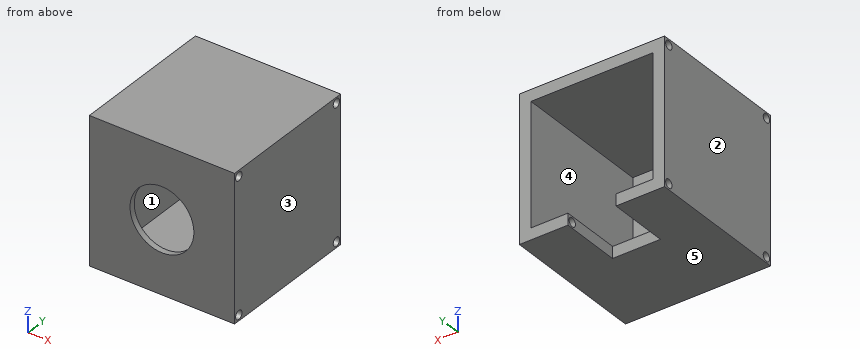
Autodesk Inventor part; units mm, degrees
ref_plane "YZ Plane" through (0, 0, 0) normal (1, 0, 0) x (0, 1, 0)
ref_plane "XZ Plane" through (0, 0, 0) normal (0, 1, 0) x (-1, 0, 0)
ref_plane "XY Plane" through (0, 0, 0) normal (0, 0, 1) x (1, 0, 0)
sketch "Sketch1" plane through (0, 0, 0) normal (0, 0, 1) x (1, 0, 0)
  line L0 (-25, -25) -> (25, -25)
  line L1 (25, -25) -> (25, 25)
  line L2 (25, 25) -> (-25, 25)
  line L3 (-25, 25) -> (-25, -25)
  line L4 (-25, -25) -> (25, 25) construction
  line L5 (25, -25) -> (-25, 25) construction
  point P0 (0, 0)
  dimension "d0" = 50
  dimension "d1" = 50
extrude "Main Block" add sketch "Sketch1" along normal blind 50
sketch "Sketch2" plane through (-25, 25, 0) normal (0, 1, 0) x (1, 0, 0)
  line L0 (0, -50) -> (50, -50) construction
  line L1 (0, 0) -> (50, 0) construction
  line L2 (50, -50) -> (0, 0) construction
  line L3 (46, -46) -> (4, -46)
  line L4 (4, -46) -> (4, -4)
  line L5 (4, -4) -> (46, -4)
  line L6 (46, -4) -> (46, -46)
  line L7 (46, -46) -> (4, -4) construction
  line L8 (4, -46) -> (46, -4) construction
  line L9 (25, -25) -> (25, -46) construction
  point P0 (25, 0)
  dimension "d4" = 42
  dimension "d5" = 42
extrude "Motor Void" cut sketch "Sketch2" against normal blind 48
sketch "Sketch3" plane through (-25, 25, 0) normal (0, 1, 0) x (1, 0, 0)
  line L0 (25, 0) -> (25, -4) construction
  line L1 (4, -4) -> (46, -4) construction
  line L2 (16.75, -4) -> (33.25, -4)
  line L3 (33.25, -4) -> (33.25, 0)
  line L4 (33.25, 0) -> (16.75, 0)
  line L5 (16.75, 0) -> (16.75, -4)
  line L6 (16.75, -4) -> (33.25, 0) construction
  line L7 (33.25, -4) -> (16.75, 0) construction
  point P0 (25, -2)
  dimension "d8" = 16.5
  dimension "d9" = 4
extrude "Cable Void" cut sketch "Sketch3" against normal blind 21
sketch "Sketch4" plane through (-25, -25, 0) normal (0, -1, 0) x (1, 0, 0)
  line L0 (0, 0) -> (0, 50) construction
  line L1 (50, 50) -> (0, 50) construction
  line L2 (0, 0) -> (50, 50) construction
  circle A0 centre (25, 25) radius 11
  point P0 (25, 0)
  dimension "d12" = 22
extrude "Raised Void" cut sketch "Sketch4" against normal blind 2
sketch "Sketch5" plane through (-25, -25, 0) normal (-1, 0, 0) x (0, 0, 1)
  line L0 (0, 0) -> (0, 50) construction
  line L1 (4, 50) -> (4, 2) construction
  line L2 (0, 50) -> (4, 50) construction
  line L3 (0, 50) -> (50, 50) construction
  line L4 (46, 2) -> (4, 2) construction
  line L5 (4, 50) -> (4, 2) construction
  line L6 (4, 2) -> (46, 2) construction
  line L7 (46, 50) -> (46, 2) construction
  line L8 (46, 2) -> (46, 50) construction
  line L9 (50, 0) -> (50, 50) construction
  line L10 (46, 50) -> (50, 50) construction
  line L11 (50, 50) -> (48, 50) construction
  line L12 (48, 50) -> (48, 48) construction
  circle A0 centre (48, 48) radius 1.5
  line L13 (48, 0) -> (48, 2) construction
  line L14 (48, 0) -> (50, 0) construction
  line L15 (0, 50) -> (4, 50) construction
  line L16 (2, 50) -> (2, 48) construction
  line L17 (0, 0) -> (50, 0) construction
  line L18 (2, 0) -> (2, 2) construction
  line L19 (2, 0) -> (4, 0) construction
  circle A1 centre (2, 48) radius 1.5
  circle A2 centre (2, 2) radius 1.5
  circle A3 centre (48, 2) radius 1.5
  point P0 (0, 25)
  dimension "d15" = 2
  dimension "d16" = 3
  dimension "d17" = 2
  dimension "d18" = 90
  dimension "d19" = 2
  dimension "d20" = 2
  dimension "d21" = 90
  dimension "d22" = 3
  dimension "d23" = 3
  dimension "d24" = 3
  dimension "d25" = 2
  dimension "d26" = 48
  dimension "d27" = 2
extrude "Extrusion5" cut sketch "Sketch5" against normal blind 50
properties part number "50x50Motor"
The listing builds one solid part. Answer for the finished solid, in the listing's coordinates (mm). Face numbers are marked on the shaded views. A direction names the side the tool comes from. Coordinates: 2 decimals unless noted, no trailing zeros. Order: outer loops, then holes, each group sorted by start corner. A loop starts at its lowest first (then second) coordinate and runs counter-clockwise, first axis right, second up.
Q1. Which of the six approach directions +Z, -Z, +X, -X, +Y, -Y give full straight-line access (tool end or side, diameter ignored) to the marked faces 1 and 2?
Q2. A cutting plane is placed at D-D, the plane z = 25. Write down the section's boundary in (x, y), and give its area (3 significant figures).
Q3. A cutting plane is placed at B-B, the plane x = 0. Write down the section's boundary in (y, z), and give its area (3 significant figures).
Q4. Consider line 1 (Y direction, x = 21, z = 2); line 2 (X direction, y = -5, z = 24); line 3 (Z direction, x = 5, y = -1). Determine where each line is inside the solid, lowest interval first.
Q5. A cutting plane is placed at A-A, the plane z = 48. Write down the section's boundary in (x, y), and give its area (3 significant figures).
Q6. A cutting plane is placed at C-C, the plane y = 23. Write down the section's boundary in (x, z).
Q7. For a pull along Z with two mould halves and no side action, classify the marked faces 3, 4 and 5 as pulls with the +Z half, pulls with the -Z half, needs draft (parallel to the pull), parting line crosses it, or undercut.
Q8. Given P1, Ø20, axis at x = 0, z = 25, coming from the -Y side; P2, Ø4.5, axis at x = -3.5, z = 1.5, coming from the +Y side; P3, Ø21, axis at x = 9, z = 26, coming from the +Y side; P4, Ø10, axis at x = 0, y = 18, coming from the -Z side, each flat-ended and moving along its own axis, determine where each tip first touches the part or whether it passes through.
Answers follow:
1. face 1: +Y
1. face 2: +Z, -Z, -X, +Y, -Y
2. outline: (-25, -25) - (-11, -25) - (-11, -23) - (-21, -23) - (-21, 25) - (-25, 25) - close; (11, -25) - (25, -25) - (25, 25) - (21, 25) - (21, -23) - (11, -23) - close
2. area: 440 mm2
3. outline: (-25, 0) - (4, 0) - (4, 4) - (-23, 4) - (-23, 14) - (-25, 14) - close; (-25, 36) - (-23, 36) - (-23, 46) - (25, 46) - (25, 50) - (-25, 50) - close; hole circle Ø3 at (-23, 2); hole circle Ø3 at (-23, 48); hole circle Ø3 at (23, 48)
3. area: 335 mm2
4. line 1: y = -25 to -24.5, -21.5 to 21.5, 24.5 to 25
4. line 2: x = -25 to -21, 21 to 25
4. line 3: z = 0 to 4, 46 to 50
5. outline: (-25, -25) - (25, -25) - (25, -24.5) - (-25, -24.5) - close; (-25, -21.5) - (25, -21.5) - (25, 21.5) - (-25, 21.5) - close; (-25, 24.5) - (25, 24.5) - (25, 25) - (-25, 25) - close
5. area: 2,200 mm2
6. outline: (-25, 0) - (-8.25, 0) - (-8.25, 0.5) - (-25, 0.5) - close; (-25, 3.5) - (-8.25, 3.5) - (-8.25, 4) - (-21, 4) - (-21, 46) - (21, 46) - (21, 4) - (8.25, 4) - (8.25, 3.5) - (25, 3.5) - (25, 46.5) - (-25, 46.5) - close; (-25, 49.5) - (25, 49.5) - (25, 50) - (-25, 50) - close; (8.25, 0) - (25, 0) - (25, 0.5) - (8.25, 0.5) - close
7. face 3: needs draft
7. face 4: undercut
7. face 5: pulls with the -Z half
8. P1: passes through
8. P2: stops at y = 4
8. P3: stops at y = -23
8. P4: stops at z = 46
